For this review, take the finished solid that the model builds, in its own axes (mm). Face numbers are marked on the shaded views. Give positions to 0.01 mm unless a question says otherwise; leave off trailing zeros. Order: outer loops, then holes, each group sorted by start corner. A loop starts at its lowest first (then second) coordinate and runs counter-clockwise, first axis right, second up.
Item 1: The part is to be moulded in two halves that separate along Y. For the marked faces 1, 2 and 3, say which applies: released by +Y, released by -Y, zero draft, split by the parting line, or undercut.
Item 2: For P1, Ø6, axis at x = 2.5, y = 4.5, coming from the -Z side, flat-tipped, find the tip position at first contact; note if it passes through.
Item 3: Consider section B-B (x = 0). Give the boundary of the cut face in (y, z) (3 decimals), plus the area to 3 significant figures.
Item 4: Consider section D-D (x = 6.75). Give the boundary of the cut face in (y, z).
Item 5: For probe 1 along X at (y, z) = (-1.5, 1.15); probe 2 along Y at (x, z) = (-0.25, 4.4); probe 3 along X at (y, z) = (4, 2.45), list the stretches that pass through material, from the lowest coordinate up.
Item 6: Consider section C-C (z = 3.9). Give the boundary of the cut face in (x, y) (3 decimals), plus the area to 3 significant figures.
Item 7: Consider section A-A (y = 0). Give the boundary of the cut face in (x, z) (3 decimals), plus the area to 3 significant figures.
```python
from build123d import *

# Parameters (mm, degrees)
SKETCH1_R           = 7.625014315
SKETCH1_R_2         = 5.125
BOSS_EXTRUDE1_DEPTH = 5
FILLET1_R           = 4


with BuildPart() as part:
    # Sketch1 → Boss-Extrude1 (new body)
    # profile 1 of 3: a face of its own
    with BuildSketch(Plane.XY):
        Circle(SKETCH1_R)
        Circle(SKETCH1_R_2, mode=Mode.SUBTRACT)
    # profile 2 of 3: a face of its own
    with BuildSketch(Plane.XY):
        with BuildLine():
            ThreePointArc((-7.178939445, 2.56976103), (-4.390124068, 6.234392831), (0, 7.625014315))
            Line((0, 7.625014315), (0, 22.625))
            Line((0, 22.625), (-7.178939445, 2.56976103))
        make_face()
    # profile 3 of 3: a face of its own
    with BuildSketch(Plane.XY):
        with BuildLine():
            Line((0, 22.625), (0, 7.625014315))
            ThreePointArc((0, 7.625014315), (4.390124068, 6.234392831), (7.178939445, 2.56976103))
            Line((7.178939445, 2.56976103), (0, 22.625))
        make_face()
    extrude(amount=BOSS_EXTRUDE1_DEPTH)

    # Fillet1
    fillet1_edges = [part.edges().sort_by_distance(p)[0] for p in [
        (0, 22.625, 2.5),
    ]]
    fillet(fillet1_edges, radius=FILLET1_R)


solid = part.part
```
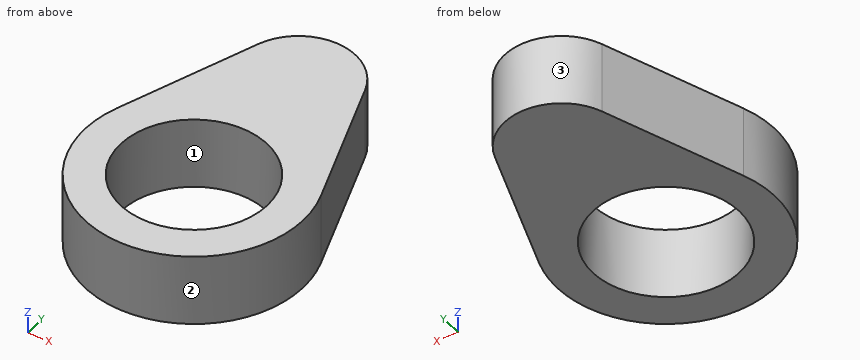
Resolved:
1. face 1: undercut
1. face 2: split by the parting line
1. face 3: released by +Y
2. P1: stops at z = 0
3. outline: (-7.625, 0) - (-5.125, 0) - (-5.125, 5) - (-7.625, 5) - close; (5.125, 0) - (14.756, 0) - (14.756, 5) - (5.125, 5) - close
3. area: 60.7 mm2
4. outline: (-3.55, 0) - (3.77, 0) - (3.77, 5) - (-3.55, 5) - close
5. probe 1: x = -7.48 to -4.9, 4.9 to 7.48
5. probe 2: y = -7.62 to -5.12, 5.12 to 14.75
5. probe 3: x = -6.67 to -3.2, 3.2 to 6.67
6. outline: (-7.179, 2.57) arc R7.625 ccw (long way) to (7.179, 2.57) - (3.766, 12.104) arc R4 ccw to (-3.766, 12.104) - close; hole circle Ø10.25 at (0, 0)
6. area: 166 mm2
7. outline: (-7.625, 0) - (-5.125, 0) - (-5.125, 5) - (-7.625, 5) - close; (5.125, 0) - (7.625, 0) - (7.625, 5) - (5.125, 5) - close
7. area: 25.0 mm2
